from build123d import *

# Parameters (mm, degrees)
SKETCH1_W            = 101.6
SKETCH1_H            = 50.8
BASE_FLANGE1_DEPTH   = 2.54
EDGE_FLANGE1_DEPTH   = 101.6
EDGE_FLANGE2_START   = -50.8
EDGE_FLANGE2_DEPTH   = 101.6
EDGE_FLANGE2_2_DEPTH = 101.6
SKETCH12_R           = 2.38125
CUT_EXTRUDE1_DEPTH   = 130.341409222


# Read off the part's stored shape, not the designer's step: Edge-Flange2
# Sheet-metal steps are written as plain solids
with BuildPart() as part:
    # Sketch1 → Base-Flange1 (new body)
    with BuildSketch(Plane.XY):
        Rectangle(SKETCH1_W, SKETCH1_H)
    extrude(amount=-BASE_FLANGE1_DEPTH)

    # Edge-Flange1 section (across the edge) → Edge-Flange1 (add)
    with BuildSketch(Plane(origin=(50.8, -25.519501076, -2.54), x_dir=(0, 0.3161458239738, -0.9487106081329159), z_dir=(-1, 0, 0))):
        with BuildLine():
            Line((-2.54, 0.119501076), (-2.54, 85.312927325))
            Line((-2.54, 85.312927325), (0, 85.312927325))
            Line((0, 85.312927325), (0, 0.119501076))
            ThreePointArc((0, 0.119501076), (0.009506284, 0.001542236), (0.037779766, -0.113371938))
            Line((0.037779766, -0.113371938), (-2.371945179, -0.916382331))
            ThreePointArc((-2.371945179, -0.916382331), (-2.497713427, -0.405212383), (-2.54, 0.119501076))
        make_face()
    extrude(amount=EDGE_FLANGE1_DEPTH)

    # Edge-Flange2 outline → Edge-Flange2 (cut)
    with BuildSketch(Plane.YZ.offset(EDGE_FLANGE2_START)):
        with BuildLine():
            Line((-106.45678024, -29.511325705), (-106.45024051, -29.136664838))
            ThreePointArc((-106.45024051, -29.136664838), (-105.815351907, -27.254750412), (-104.210022959, -26.085304214))
            Line((-104.210022959, -26.085304214), (-107.259790633, -27.10160076))
            Line((-107.259790633, -27.10160076), (-106.45678024, -29.511325705))
        make_face()
    extrude(amount=EDGE_FLANGE2_DEPTH, mode=Mode.SUBTRACT)

    # Edge-Flange2 2 outline → Edge-Flange2 2 (add)
    with BuildSketch(Plane.YZ.offset(EDGE_FLANGE2_START)):
        with BuildLine():
            Line((-103.407012566, -28.495029159), (-106.45678024, -29.511325705))
            Line((-106.45678024, -29.511325705), (-106.853065184, -52.214474934))
            Line((-106.853065184, -52.214474934), (-104.313452038, -52.258804046))
            Line((-104.313452038, -52.258804046), (-103.910627364, -29.18099395))
            ThreePointArc((-103.910627364, -29.18099395), (-103.767900469, -28.757927917), (-103.407012566, -28.495029159))
        make_face()
    extrude(amount=EDGE_FLANGE2_2_DEPTH)

    # Sketch12 → Cut-Extrude1 (cut, through all)
    with BuildSketch(Plane.XY):
        with Locations((-25.4, 12.7)):
            Circle(SKETCH12_R)
        with Locations((0, 12.7)):
            Circle(SKETCH12_R)
        with Locations((25.4, 12.7)):
            Circle(SKETCH12_R)
        with Locations((25.4, -12.7)):
            Circle(SKETCH12_R)
        with Locations((0, -12.7)):
            Circle(SKETCH12_R)
        with Locations((-25.4, -12.7)):
            Circle(SKETCH12_R)
    extrude(amount=-CUT_EXTRUDE1_DEPTH, mode=Mode.SUBTRACT)


solid = part.part
Read the model definition and answer for the solid it produces. Units are mm, in the model's axes. Coordinates: 2 decimals unless noted, no trailing zeros. Loops run counter-clockwise (first coordinate to the right, second up) from the corner with the lowest first, then second, coordinate; pieces in that order, holes last. Notation, with made-up numbers: (-4.5, -6) -> (40.5, -6) arc R35 ccw to (40.5, 33) -> close; hole circle Ø10 at (39.25, 31). An arc over 180 degrees is marked (long way). Write item = value, one per line. Start each with the question number.
1) The part is cut by section B-B, the plane y = 12.7. Determine the outline of the cut face in (x, z), plus the area to 3 significant figures.
2) The part is cut by section C-C, the plane x = 17. Determine the outline of the cut face in (y, z), plus the area to 3 significant figures.
3) The mould has two halves that part along X. Classify faces 1 (the face through (23.645, -11.091, -1.252)), 2 (the face through (50.8, -61, -12)), 3 (the face through (-1, 0, -2.54)): pulls with the +X half, pulls with the -X half, needs draft (parallel to the pull), parting line crosses it, or undercut.
4) Given P1, Ø1, axis at x = 38.5, z = -26, coming from the -Y side; P2, Ø12, axis at x = -22.5, z = -47, coming from the +Y side; P3, Ø5, axis at x = 35, y = -31, coming from the +Z side, each flat-ended and moving along its own axis, determine where each tip first touches the part or whether it passes through.
5) The part is cut by section D-D, the plane y = -72. Determine the outline of the cut face in (x, z).
6) The part is cut by section A-A, the plane x = 0. Determine the outline of the cut face in (y, z).
7) Find the intervals of material crossed by L1, parallel to X at y = 12, z = -1; L2, parallel to Z at x = 44, y = -1; L3, parallel to Y at x = 42.5, z = -46, in increasing order. Write a range as from..to.
Result:
q1.outline = (-50.8, -2.54) -> (-27.78, -2.54) -> (-27.78, 0) -> (-50.8, 0) -> close; (-23.02, -2.54) -> (-2.38, -2.54) -> (-2.38, 0) -> (-23.02, 0) -> close; (2.38, -2.54) -> (23.02, -2.54) -> (23.02, 0) -> (2.38, 0) -> close; (27.78, -2.54) -> (50.8, -2.54) -> (50.8, 0) -> (27.78, 0) -> close
q1.area = 222 mm²
q2.outline = (-106.85, -52.21) -> (-104.31, -52.26) -> (-103.91, -29.18) arc R0.74 cw to (-103.41, -28.5) -> (-25.63, -2.58) arc R0.74 cw to (-25.4, -2.54) -> (25.4, -2.54) -> (25.4, 0) -> (-25.4, 0) arc R3.28 ccw to (-26.44, -0.17) -> (-104.21, -26.09) arc R3.28 ccw to (-106.45, -29.14) -> close
q2.area = 404 mm²
q3.face_1 = undercut
q3.face_2 = pulls with the +X half
q3.face_3 = needs draft
q4.P1 = -105.04
q4.P2 = -104.12
q4.P3 = -0.86
q5.outline = (-50.8, -18.03) -> (50.8, -18.03) -> (50.8, -15.35) -> (-50.8, -15.35) -> close
q6.outline = (-106.85, -52.21) -> (-104.31, -52.26) -> (-103.91, -29.18) arc R0.74 cw to (-103.41, -28.5) -> (-25.63, -2.58) arc R0.74 cw to (-25.4, -2.54) -> (-15.08, -2.54) -> (-15.08, 0) -> (-25.4, 0) arc R3.28 ccw to (-26.44, -0.17) -> (-104.21, -26.09) arc R3.28 ccw to (-106.45, -29.14) -> close; (-10.32, -2.54) -> (10.32, -2.54) -> (10.32, 0) -> (-10.32, 0) -> close; (15.08, -2.54) -> (25.4, -2.54) -> (25.4, 0) -> (15.08, 0) -> close
q7.L1 = -50.8..-27.68, -23.12..-2.28, 2.28..23.12, 27.68..50.8
q7.L2 = -2.54..0
q7.L3 = -106.74..-104.2
